Here's how the part is built. I have some questions about the finished solid (model axes, mm). A direction names the side the tool comes from. Coordinates: 2 decimals unless noted, no trailing zeros. Write each loop counter-clockwise with the first axis right and the second up, starting at its lowest first coordinate (ties: lowest second). Pieces come first, ordered by that corner, then holes. Notation, with made-up numbers: M 85,1.25 L 101,1.25 A17 cw 101,27.25 Z; hole C 53.25,70.25 d4. An arc over 180 degrees is marked long. Use one line per item in the form item = value. Start each with the question number.
1. I want a section at D-D, the plane z = 6.75. Count the separate pieces of the cut face and the enclosed holes in it, plus the area to 3 significant figures.
2. Thinking about a two-plate mould opening in X: for faces 1 (the face through (10, -1, 1.5)), 2 (the face through (12.28, -3.455, 5.937)), 3 (the face through (0, 8, 6)), which applies, released by +X, released by -X, zero draft, split by the parting line, or undercut?
3. I want a section at C-C, the plane x = 5. List the corners of the cut face in (y, z) for me.
4. I want a section at B-B, the plane y = 1. List the corners of the cut face in (x, z) for me, plus the area to 3 significant figures.
5. Please list where these lines run through material, in increasing order: line 1 along Z through (x, y) = (10, 2.75); line 2 along Y through (x, z) = (8, 14.25); line 3 along Y through (x, z) = (5.25, 12.25). Write a range as [from, to].
6. I want a section at A-A, the plane z = -2. List the corners of the cut face in (x, y) for me.
7. I'm going to push flat-ended pins straight in: pin 1 Ø1.5 at (x, z) = (11.5, 3) entering from -Y; pin 2 Ø2 at (x, z) = (6, -0.5) entering from -Y; pin 3 Ø1.5 at (y, z) = (12.5, -1) entering from +X. Where does each tip first touch, or does it pass through?
8. On a 3-axis mill with a long thin cutter (end or side, diameter ignored), from which of +Z, -Z, +X, -X, +Y, -Y can I reach the whole of each face in a straight line? I mean faces 4 (the face through (4.89, 5.852, 13.479)), 5 (the face through (10, -1, 10.5)), 6 (the face through (10, 13, -2)). Say none if no direction works.
from build123d import *

# Parameters (mm, degrees)
SKETCHDISTALINTERNAL_R          = 0.5
BOSSEXTRUDEDISTALINTERNAL_DEPTH = 12
CUTEXTRUDEDISTALBARL_START      = -1.5
CUTEXTRUDEDISTALBARL_DEPTH      = 1.5
CUTEXTRUDEDISTALBARR_DEPTH      = 1.5
BOSSEXTRUDEEXTERNAL_START       = -16
BOSSEXTRUDEEXTERNAL_DEPTH       = 20
FILLETDISTALEXTERNAL_R          = 1


with BuildPart() as part:
    # SketchDistalInternal → BossExtrudeDistalInternal (new body)
    with BuildSketch(Plane.XY):
        with BuildLine():
            Line((0.839496756, -1.48710509), (11.016133562, -6.51289491))
            ThreePointArc((11.016133562, -6.51289491), (15.358517882, -5.771641109), (16, -1.4134007))
            Line((16, -1.4134007), (12.527091293, 5.230590272))
            add(Edge.make_bspline(
                [(10, 16), (10, 11.295651098), (10.473683301, 9.158946966), (12.527091293, 5.230590272)],
                knots=[0, 0, 0, 0, 1, 1, 1, 1], degree=3))
            ThreePointArc((10, 16), (5, 21), (0, 16))
            Line((0, 16), (0, 0))
            add(Edge.make_bspline(
                [(0, 0), (0, -0.54020277), (0.191605084, -1.167140113), (0.839496756, -1.48710509)],
                knots=[0, 0, 0, 0, 1, 1, 1, 1], degree=3))
        make_face()
        with Locations((2.5, 1.875219846)):
            Circle(SKETCHDISTALINTERNAL_R, mode=Mode.SUBTRACT)
        with Locations((12.676636807, -3.150569974)):
            Circle(SKETCHDISTALINTERNAL_R, mode=Mode.SUBTRACT)
    extrude(amount=BOSSEXTRUDEDISTALINTERNAL_DEPTH)

    # SketchCutBarL → CutExtrudeDistalBarL (cut)
    with BuildSketch(Plane.XY.offset(12).offset(CUTEXTRUDEDISTALBARL_START)):
        with BuildLine():
            Line((3.880618629, -2.98898038), (11.016133562, -6.51289491))
            ThreePointArc((11.016133562, -6.51289491), (15.358517882, -5.771641109), (16, -1.4134007))
            Line((16, -1.4134007), (12.527091293, 5.230590272))
            ThreePointArc((12.527091293, 5.230590272), (6.43792312, 2.978454456), (3.880618629, -2.98898038))
        make_face()
    extrude(amount=CUTEXTRUDEDISTALBARL_DEPTH, mode=Mode.SUBTRACT)

    # SketchCutBarR → CutExtrudeDistalBarR (cut)
    with BuildSketch(Plane.XY):
        with BuildLine():
            Line((3.880618629, -2.98898038), (11.016133562, -6.51289491))
            ThreePointArc((11.016133562, -6.51289491), (15.358517882, -5.771641109), (16, -1.4134007))
            Line((16, -1.4134007), (12.527091293, 5.230590272))
            ThreePointArc((12.527091293, 5.230590272), (6.43792312, 2.978454456), (3.880618629, -2.98898038))
        make_face()
    extrude(amount=CUTEXTRUDEDISTALBARR_DEPTH, mode=Mode.SUBTRACT)

    # SketchDistalExternal → BossExtrudeExternal (add)
    with BuildSketch(Plane.XY.offset(12).offset(BOSSEXTRUDEEXTERNAL_START)):
        with BuildLine():
            Line((0, 16), (0, 10.850906929))
            ThreePointArc((0, 10.850906929), (5, 5.850906929), (10, 10.850906929))
            Line((10, 10.850906929), (10, 16))
            ThreePointArc((10, 16), (5, 21), (0, 16))
        make_face()
    extrude(amount=BOSSEXTRUDEEXTERNAL_DEPTH)

    # FilletDistalExternal
    filletdistalexternal_edges = [part.edges().sort_by_distance(p)[0] for p in [
        (5, 21, -4),
        (10, 13.425453465, -4),
        (5, 5.850906929, -4),
        (0, 13.425453465, -4),
        (5, 21, 16),
        (0, 13.425453465, 16),
        (5, 5.850906929, 16),
        (10, 13.425453465, 16),
    ]]
    fillet(filletdistalexternal_edges, radius=FILLETDISTALEXTERNAL_R)


solid = part.part
Answer list:
q1.separate_pieces = 1
q1.enclosed_holes = 2
q1.area = 300 mm²
q2.face_1 = zero draft
q2.face_2 = undercut
q2.face_3 = released by -X
q3.outline = M -3.54,1.5 L 1.16,1.5 L 1.16,0 L 5.85,0 L 5.85,-3 A1 ccw 6.85,-4 L 20,-4 A1 ccw 21,-3 L 21,15 A1 ccw 20,16 L 6.85,16 A1 ccw 5.85,15 L 5.85,12 L 1.16,12 L 1.16,10.5 L -3.54,10.5 Z
q4.outline = M 0,0 L 4.91,0 L 4.91,1.5 L 14.74,1.5 L 14.74,10.5 L 4.91,10.5 L 4.91,12 L 0,12 Z
q4.area = 147 mm²
q5.line_1 = [1.5, 10.5]
q5.line_2 = [6.85, 20]
q5.line_3 = [5.86, 20.99]
q6.outline = M 0,10.85 A5 ccw 10,10.85 L 10,16 A5 ccw 0,16 Z
q7.pin_1 = -6.88
q7.pin_2 = 1.38
q7.pin_3 = 10
q8.face_4 = +Z, -Y
q8.face_5 = +Z, +X, -Y
q8.face_6 = -Z, +X, +Y, -Y
